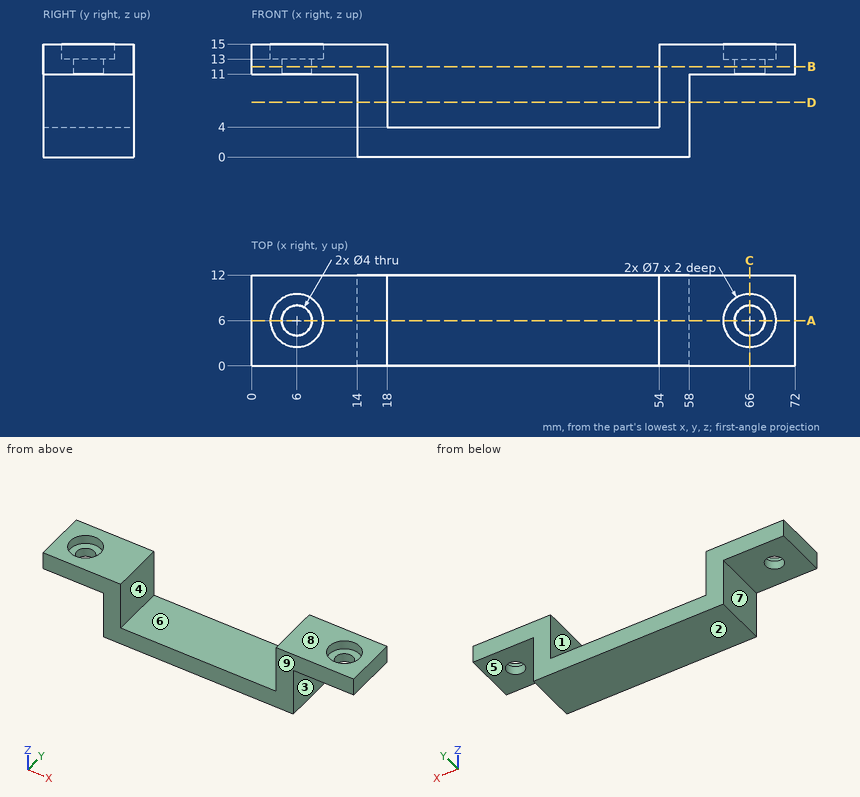
The figure shows three views and two pictorial views of one solid part (mm, origin at its lowest corner). Answer the questions. A direction names the side the tool comes from. Give positions to 0.01 mm unless a question says otherwise; leave off trailing zeros. Write each loop counter-clockwise with the first axis right and the second up, starting at its lowest first coordinate (ties: lowest second). Pieces come first, ordered by that corner, then holes. Notation, with made-up numbers: (19, -20.75) - (67, -20.75) arc R32 cw to (67, 10.25) - close; hole circle Ø7 at (89, 85.5). An arc over 180 degrees is marked (long way). Use one line per item in the form item = value.
1. A cutting plane is placed at D-D (z = 7.25). Write down the section's boundary in (x, y), and give its area (3 significant figures).
Filled in:
outline = (14, 0) - (18, 0) - (18, 12) - (14, 12) - close; (54, 0) - (58, 0) - (58, 12) - (54, 12) - close
area = 96.0 mm^2
2. Consider L1, parallel to X at y = 5, z = 5.25; L2, parallel to Y at x = 6, z = 14.65; L3, parallel to Z at x = 61, y = 6.25. Determine where each line is inside the solid, lowest interval first.
Filled in:
L1 = 14 to 18, 54 to 58
L2 = 0 to 2.5, 9.5 to 12
L3 = 11 to 15
3. A cutting plane is placed at A-A (y = 6). Write down the section's boundary in (x, z), and give its area (3 significant figures).
Filled in:
outline = (0, 11) - (4, 11) - (4, 13) - (2.5, 13) - (2.5, 15) - (0, 15) - close; (8, 11) - (14, 11) - (14, 0) - (58, 0) - (58, 11) - (64, 11) - (64, 13) - (62.5, 13) - (62.5, 15) - (54, 15) - (54, 4) - (18, 4) - (18, 15) - (9.5, 15) - (9.5, 13) - (8, 13) - close; (68, 11) - (72, 11) - (72, 15) - (69.5, 15) - (69.5, 13) - (68, 13) - close
area = 332 mm^2
4. A cutting plane is placed at B-B (z = 12). Write down the section's boundary in (x, y).
Filled in:
outline = (0, 0) - (18, 0) - (18, 12) - (0, 12) - close; (54, 0) - (72, 0) - (72, 12) - (54, 12) - close; hole circle Ø4 at (6, 6); hole circle Ø4 at (66, 6)
5. Determine the mould class of the marked faces 1, 2, 3 and 4 for opening direction X: released by +X, released by -X, zero draft, split by the parting line, or undercut.
Filled in:
face_1 = undercut
face_2 = zero draft
face_3 = released by +X
face_4 = undercut
6. Each of these flat-tipped pins is pushed along its axis until it touches: pin 1 Ø5 at (x, y) = (66, 6) entering from +Z; pin 2 Ø3 at (y, z) = (10, 2) entering from +X; pin 3 Ø5 at (x, y) = (6, 6) entering from -Z; pin 4 Ø3 at (x, z) = (47, 6.5) entering from -Y. Where does it stop, or does it pass through?
Filled in:
pin_1 = 13
pin_2 = 58
pin_3 = 11
pin_4 = through
7. A cutting plane is placed at C-C (x = 66). Write down the section's boundary in (y, z).
Filled in:
outline = (0, 11) - (4, 11) - (4, 13) - (2.5, 13) - (2.5, 15) - (0, 15) - close; (8, 11) - (12, 11) - (12, 15) - (9.5, 15) - (9.5, 13) - (8, 13) - close
8. For the marked faces 5, 6, 7, 8 and 9, determine the directions among +Z, -Z, +X, -X, +Y, -Y from which every point of the face is accessible in a straight line to the end or side of a thin tool.
Filled in:
face_5 = -Z, +X, +Y, -Y
face_6 = +Z, +Y, -Y
face_7 = -Z, -X, +Y, -Y
face_8 = +Z, +X, -X, +Y, -Y
face_9 = +Z, -Z, +X, -X, -Y
